```python
from build123d import *
from build123d.topology import SkipClean

# Parameters (mm, degrees)
BOSS_EXTRUDE1_DEPTH     = 50.8
SKETCH2_R               = 2.25
SKETCH2_R_2             = 2.2500000000000004
SKETCH2_R_3             = 2.2499999999999964
SKETCH2_R_4             = 2.250000000000002
CUT_EXTRUDE2_DEPTH      = 80.4629164554471
CUT_EXTRUDE4_DEPTH      = 80.4629164554471
CUT_EXTRUDE4_DEPTH_BACK = 80.4629164554471
SKETCH7_W               = 34.34264107490862
SKETCH7_H               = 6.349999999999994
SKETCH7_H_2             = 25.4
SKETCH7_W_2             = 12.699999999999996
BOSS_EXTRUDE3_START     = 12.7
BOSS_EXTRUDE3_DEPTH     = 34.342641075
CUT_EXTRUDE5_DEPTH      = 81.46127057538526
CUT_EXTRUDE5_DEPTH_BACK = 81.46127057538526
CAVITY1_START           = -12.110223167
CAVITY1_DEPTH           = 25.933177896
CHAMFER5_SIZE           = 2.54


with BuildPart() as part:
    # Sketch1 → Boss-Extrude1 (new body)
    with BuildSketch(Plane.XY):
        with BuildLine():
            Line((0, 5.08), (0, 0))
            Line((0, 0), (11.964320537454306, 0))
            ThreePointArc((11.964320537454306, 2.19e-15), (12.149194735731278, 2.56649684743677), (12.700000000000003, 5.080000000000005))
            Line((12.7, 5.08), (0, 5.08))
        make_face()
        with BuildLine():
            ThreePointArc((12.700000000000003, 5.080000000000005), (12.149194735731278, 2.56649684743677), (11.964320537454306, 2.19e-15))
            Line((11.964320537454306, 0), (17.044320537454304, 0))
            ThreePointArc((17.044320537454304, 1.57e-15), (20.80126185517433, 9.070058682279722), (29.871320537453954, 12.827000000000004))
            Line((29.871320537454306, 12.827000000000004), (29.871320537454306, 17.907))
            ThreePointArc((29.871320537454306, 17.907), (19.154672530731307, 14.34622265615587), (12.700000000000003, 5.080000000000005))
        make_face()
        with BuildLine():
            Line((42.69832053745431, 0), (47.778320537454306, 0))
            ThreePointArc((47.778320537454306, 0), (47.59344633917733, 2.56649684743677), (47.042641074908616, 5.079999999999999))
            ThreePointArc((47.042641074908616, 5.079999999999999), (40.5879685441773, 14.34622265615587), (29.871320537454306, 17.907))
            Line((29.871320537454306, 17.907), (29.871320537454306, 12.827000000000004))
            ThreePointArc((29.871320537453954, 12.827000000000004), (38.94137921973403, 9.070058682279972), (42.69832053745431, 0))
        make_face()
        with BuildLine():
            ThreePointArc((47.042641074908616, 5.079999999999999), (47.59344633917733, 2.56649684743677), (47.778320537454306, 0))
            Line((47.778320537454306, 0), (59.74264107490861, 0))
            Line((59.74264107490861, 0), (59.74264107490861, 5.08))
            Line((59.74264107490861, 5.08), (47.042641074908616, 5.08))
        make_face()
    extrude(amount=BOSS_EXTRUDE1_DEPTH)

    # Sketch2 → Cut-Extrude2 (cut, through all)
    with BuildSketch(Plane(origin=(0, 5.08, 0), x_dir=(1, 0, 0), z_dir=(0, 1, 0))):
        with Locations(Location((6.349999999999999, -12.7, 0), (0, 0, 270))):
            Circle(SKETCH2_R)
        with Locations(Location((6.350000000000002, -38.10000000000001, 0), (0, 0, 270))):
            Circle(SKETCH2_R_2)
        with Locations(Location((53.392641074908624, -38.1, 0), (0, 0, 270))):
            Circle(SKETCH2_R_3)
        with Locations(Location((53.39264107490862, -12.699999999999994, 0), (0, 0, 270))):
            Circle(SKETCH2_R_4)
    extrude(amount=-CUT_EXTRUDE2_DEPTH, mode=Mode.SUBTRACT)

    # Sketch7 → Cut-Extrude4 (cut, two sides: drawn at the far end of the back side and taken through both)
    with BuildSketch(Plane(origin=(0, 5.08, 0), x_dir=(1, 0, 0), z_dir=(0, 1, 0)).offset(-CUT_EXTRUDE4_DEPTH_BACK)):
        Polygon((0, -50.8), (12.700000000000001, -50.8), (12.7, -44.449999999999996), (0, -44.449999999999996), align=None)
        with Locations((29.871320537454306, -47.62499999999999)):
            Rectangle(SKETCH7_W, SKETCH7_H)
        with Locations((29.871320537454306, -31.749999999999996)):
            Rectangle(SKETCH7_W, SKETCH7_H_2)
        with Locations((53.39264107490861, -47.62499999999999)):
            Rectangle(SKETCH7_W_2, SKETCH7_H)
    extrude(amount=CUT_EXTRUDE4_DEPTH + CUT_EXTRUDE4_DEPTH_BACK, mode=Mode.SUBTRACT)

    # Sketch8 → Boss-Extrude3 (add)
    with BuildSketch(Plane(origin=(0, 0, 0), x_dir=(0, 0, -1), z_dir=(1, 0, 0)).offset(BOSS_EXTRUDE3_START)):
        Polygon((-19.049999999999997, 5.0799999999999965), (-19.049999999999994, 30.479999999999997), (0, 17.907), (0, 5.079999999999999), align=None)
    extrude(amount=BOSS_EXTRUDE3_DEPTH)

    # Sketch1<4> → Cut-Extrude5 (cut, two sides: drawn at the far end of the back side and taken through both)
    with SkipClean():  # the faces are left unmerged after this step: merging them gives an invalid solid
        with BuildSketch(Plane.XY.offset(-CUT_EXTRUDE5_DEPTH_BACK)):
            with BuildLine():
                ThreePointArc((29.871320537453954, 12.827000000000004), (20.80126185517433, 9.070058682279722), (17.044320537454304, 1.57e-15))
                Line((17.044320537454304, 0), (29.871320537454306, 0))
                Line((29.871320537454306, 0), (29.871320537454306, 12.827000000000004))
            make_face()
            with BuildLine():
                Line((29.871320537454306, 0), (17.044320537454304, 0))
                ThreePointArc((17.044320537454304, 1.57e-15), (29.871320537454302, -12.827000000000004), (42.69832053745431, -3.14e-15))
                ThreePointArc((42.69832053745431, 0), (38.94137921973403, 9.070058682279972), (29.871320537453954, 12.827000000000004))
                Line((29.871320537454306, 12.827000000000004), (29.871320537454306, 0))
            make_face()
        extrude(amount=CUT_EXTRUDE5_DEPTH + CUT_EXTRUDE5_DEPTH_BACK, mode=Mode.SUBTRACT)

    # Cavity1: read off the stored shape, not the designer's step
    # Cavity1 outline → Cavity1 (cut)
    with SkipClean():  # the faces are left unmerged after this step: merging them gives an invalid solid
        with BuildSketch(Plane(origin=(0, 0, 0), x_dir=(1, 0, 0), z_dir=(0, 0.7719302356170498, -0.6357072528610997)).offset(CAVITY1_START)):
            with BuildLine():
                Line((42.335603858, -36), (41.488040544, -34.081628056))
                ThreePointArc((41.488040544, -34.081628056), (29.871320538, -26.514055969), (18.254600531, -34.081628056))
                Line((18.254600531, -34.081628056), (17.407037217, -36))
                Line((17.407037217, -36), (42.335603858, -36))
            make_face()
        extrude(amount=CAVITY1_DEPTH, mode=Mode.SUBTRACT)

    # Chamfer5
    # the kernel refuses this chamfer: 2.54 mm, written as the material it adds along each edge
    with BuildSketch(Plane(origin=(12.700000000000003, 5.080000000000004, 0), x_dir=(-1, -1.4e-15, 0), z_dir=(0, 0, 1))) as chamfer5_piece_1:
        Polygon((CHAMFER5_SIZE, 0), (0, -CHAMFER5_SIZE), (0, 0), align=None)
    extrude(amount=19.049999999999997)
    with BuildSketch(Plane(origin=(47.042641074908616, 5.08, 0), x_dir=(3.598031758927257e-11, 1.0, 0), z_dir=(0, 0, 1))) as chamfer5_piece_2:
        Polygon((CHAMFER5_SIZE, 0), (9.139001e-11, -CHAMFER5_SIZE), (0, 0), align=None)
    extrude(amount=19.049999999999997)
    # the kernel refuses this chamfer: 2.54 mm, written as the material it takes off along each edge
    with BuildSketch(Plane(origin=(42.69832053745431, -1.3e-16, -7.4053740903902145), x_dir=(1, 5e-17, 0), z_dir=(0, 0, 1))) as chamfer5_2_piece_1:
        with BuildLine():
            Line((CHAMFER5_SIZE, 0), (-0.3237705210766462, 2.863770521075717))
            ThreePointArc((-0.3237705210766462, 2.863770521075717), (-0.08576469637885246, 1.4808281256642715), (0, 0))
            Line((0, 0), (CHAMFER5_SIZE, 0))
        make_face()
    extrude(amount=33.860748180780426, mode=Mode.SUBTRACT)
    with BuildSketch(Plane(origin=(17.044320537454304, 7.9e-16, -7.405374090390225), x_dir=(0.11234172985080312, 0.9936696310817439, 0), z_dir=(0, 0, 1))) as chamfer5_2_piece_2:
        with BuildLine():
            Line((2.882014737592532, 1e-17), (-CHAMFER5_SIZE * 0.112341729851, CHAMFER5_SIZE * 0.993669631082))
            Line((-CHAMFER5_SIZE * 0.112341729851, CHAMFER5_SIZE * 0.993669631082), (0, 0))
            ThreePointArc((0, 0), (1.4810888916756169, 0.0811370190382275), (2.882014737592532, 1e-17))
        make_face()
    extrude(amount=33.86074818078045, mode=Mode.SUBTRACT)
    with BuildSketch(Plane(origin=(47.042641075000006, 34.07814250199304, 24.501731063625822), x_dir=(-1, 6.4e-16, -4.2e-16), z_dir=(0, -0.5508422083307387, -0.8346094065617252))) as chamfer5_2_piece_3:
        Polygon((CHAMFER5_SIZE, 0), (-1.96e-15, -CHAMFER5_SIZE), (0, 0), align=None)
    extrude(amount=35.889197859210064, mode=Mode.SUBTRACT)
    with BuildSketch(Plane(origin=(12.7, 34.07814250199304, 24.50173106362582), x_dir=(0, -0.8346094065617252, 0.5508422083307387), z_dir=(0, -0.5508422083307387, -0.8346094065617252))) as chamfer5_2_piece_4:
        Polygon((CHAMFER5_SIZE, 0), (0, -CHAMFER5_SIZE), (0, 0), align=None)
    extrude(amount=35.88919785921006, mode=Mode.SUBTRACT)


solid = part.part
```
Check sheet for the modelled part. Datum: model origin and axes. Units: mm. A direction names the side the tool comes from. Give positions to 0.01 mm unless a question says otherwise; leave off trailing zeros. Loops run counter-clockwise (first coordinate to the right, second up) from the corner with the lowest first, then second, coordinate; pieces in that order, holes last. Notation, with made-up numbers: M 3.25,-2.75 L 60.25,-2.75 A6 ccw 60.25,8.25 Z; hole C 51.5,57 d11. An arc over 180 degrees is marked long. Answer in a Markdown table with one row per item.
1) Tool access check on faces 5 (the face through (15.956, 1.452, 9.392)), 6 (the face through (6, 5.08, 22)), 7 (the face through (29, 13, 0)). Record the directions out of +Z, -Z, +X, -X, +Y, -Y that give a thin tool (end or side, any length) a straight path to the whole face; none if there is none.
Solutions:
| item | result |
|---|---|
| face 5 | +Z, -Z, -Y |
| face 6 | +Z, -X, +Y |
| face 7 | -Z, +X, -X, +Y, -Y |
2) Cross-section at B-B (y = 4). Enter the section's corners in (x, z).
Solutions:
| item | result |
|---|---|
| outline | M 0,0 L 17.68,0 L 17.68,19.05 L 12.7,19.05 L 12.7,44.45 L 0,44.45 Z; M 42.06,0 L 59.74,0 L 59.74,44.45 L 47.04,44.45 L 47.04,19.05 L 42.06,19.05 Z; hole C 6.35,12.7 d4.5; hole C 6.35,38.1 d4.5; hole C 53.39,12.7 d4.5; hole C 53.39,38.1 d4.5 |
3) Cross-section at D-D (z = 21). Enter the section's corners in (x, y).
Solutions:
| item | result |
|---|---|
| outline | M 0,0 L 12.7,0 L 12.7,5.08 L 0,5.08 Z; M 47.04,0 L 59.74,0 L 59.74,5.08 L 47.04,5.08 Z |
4) Thickness scan on line 1 (X direction, y = 2, z = 38.1); line 2 (X direction, y = 1, z = 26.5); line 3 (Z direction, x = 6, y = 2). Record the ranges inside material, lowest first.
Solutions:
| item | result |
|---|---|
| line 1 | x = 0 to 4.1, 8.6 to 12.7, 47.04 to 51.14, 55.64 to 59.74 |
| line 2 | x = 0 to 12.7, 47.04 to 59.74 |
| line 3 | z = 0 to 10.48, 14.92 to 35.88, 40.32 to 44.45 |
5) Cross-section at A-A (z = 38.1). Enter the section's corners in (x, y).
Solutions:
| item | result |
|---|---|
| outline | M 0,0 L 4.1,0 L 4.1,5.08 L 0,5.08 Z; M 8.6,0 L 12.7,0 L 12.7,5.08 L 8.6,5.08 Z; M 47.04,0 L 51.14,0 L 51.14,5.08 L 47.04,5.08 Z; M 55.64,0 L 59.74,0 L 59.74,5.08 L 55.64,5.08 Z |
6) Mould release check, pull along X, two halves, no side actions. Record for faces 1 (the face through (43.83, 1.41, 9.39)), 2 (the face through (6, 3, 44.45)), 3 (the face through (47.043, 3, 32)), 4 (the face through (48.29, 6.37, 9.39)): released by +X, released by -X, zero draft, split by the parting line, or undercut.
Solutions:
| item | result |
|---|---|
| face 1 | undercut |
| face 2 | zero draft |
| face 3 | undercut |
| face 4 | released by +X |
7) Cross-section at C-C (x = 6.35). Enter the section's corners in (y, z).
Solutions:
| item | result |
|---|---|
| outline | M 0,0 L 5.08,0 L 5.08,10.45 L 0,10.45 Z; M 0,14.95 L 5.08,14.95 L 5.08,35.85 L 0,35.85 Z; M 0,40.35 L 5.08,40.35 L 5.08,44.45 L 0,44.45 Z |
8) Depth check by flat-ended pin: pin 1 (2 mm diameter, centred on x = 11, y = 22.5, fed in from -Z); pin 2 (5 mm diameter, centred on x = 13, z = 8.5, fed in from +Y); pin 3 (5 mm diameter, centred on x = 45.5, y = 12, fed in from +Z); pin 4 (15 mm diameter, centred on y = 22, z = 9, fed in from +X). Enter the tip coordinate at first touch or a pass-through.
Solutions:
| item | result |
|---|---|
| pin 1 | passes through |
| pin 2 | stops at y = 24.25 |
| pin 3 | stops at z = 19.05 |
| pin 4 | stops at x = 47.04 |
